from build123d import *

# Parameters (mm, degrees)
SKETCH1_R               = 9.64479785
BOSS_EXTRUDE1_DEPTH     = 1
SKETCH2_W               = 8
SKETCH2_H               = 8
SKETCH2_W_2             = 10
SKETCH2_H_2             = 10
SKETCH2_W_3             = 7
SKETCH2_H_3             = 7
BOSS_EXTRUDE2_DEPTH     = 9.5
SKETCH3_R               = 0.9
CUT_EXTRUDE1_DEPTH      = 8
CUT_EXTRUDE2_DEPTH      = 0.7
SKETCH6_R               = 6.717749006
CUT_EXTRUDE7_DEPTH      = 10.5
CUT_EXTRUDE7_DEPTH_BACK = 2


with BuildPart() as part:
    # Sketch1 → Boss-Extrude1 (new body)
    with BuildSketch(Plane.XY):
        with BuildLine():
            Line((-14.026724751, 23.745574299), (14.026724751, 23.745574299))
            ThreePointArc((14.026724751, 23.745574299), (37.77229905, 0), (14.026724751, -23.745574299))
            Line((14.026724751, -23.745574299), (-14.026724751, -23.745574299))
            ThreePointArc((-14.026724751, -23.745574299), (-37.77229905, 0), (-14.026724751, 23.745574299))
        make_face()
        Circle(SKETCH1_R, mode=Mode.SUBTRACT)
    extrude(amount=BOSS_EXTRUDE1_DEPTH)

    # Sketch2 → Boss-Extrude2 (add)
    with BuildSketch(Plane.XY.offset(1)):
        with Locations((-25.018703454, 11.462322744)):
            Rectangle(SKETCH2_W, SKETCH2_H)
        with Locations((-3.090198121, -14.497536266)):
            Rectangle(SKETCH2_W_2, SKETCH2_H_2)
        with Locations((25.327090693, 14.846915234)):
            Rectangle(SKETCH2_W_3, SKETCH2_H_3)
    extrude(amount=BOSS_EXTRUDE2_DEPTH)

    # Sketch3 → Cut-Extrude1 (cut)
    with BuildSketch(Plane.XY.offset(10.5)):
        with Locations((-25.018703454, 11.462322744)):
            Circle(SKETCH3_R)
        with Locations((25.327090693, 14.846915234)):
            Circle(SKETCH3_R)
        with Locations((-3.090198121, -14.497536266)):
            Circle(SKETCH3_R)
    extrude(amount=-CUT_EXTRUDE1_DEPTH, mode=Mode.SUBTRACT)

    # Sketch4 → Cut-Extrude2 (cut)
    with BuildSketch(Plane.XY.offset(1)):
        with BuildLine():
            Line((-20.6, 6.2), (-36.948598558, 6.2))
            ThreePointArc((-36.948598558, 6.2), (-37.70555704, 1.779100955), (-37.617693234, -2.705273523))
            Line((-37.617693234, -2.705273523), (-20.6, -2.705273523))
            Line((-20.6, -2.705273523), (-20.6, 6.2))
        make_face()
    extrude(amount=-CUT_EXTRUDE2_DEPTH, mode=Mode.SUBTRACT)

    # Sketch6 → Cut-Extrude7 (cut, two sides)
    with BuildSketch(Plane.XY.offset(1)) as cut_extrude7_sk:
        with Locations((14.176031791, 0)):
            Circle(SKETCH6_R)
        with Locations((-14.176031791, 0)):
            Circle(SKETCH6_R)
    extrude(amount=CUT_EXTRUDE7_DEPTH, mode=Mode.SUBTRACT)
    extrude(cut_extrude7_sk.sketch, amount=-CUT_EXTRUDE7_DEPTH_BACK, mode=Mode.SUBTRACT)


solid = part.part
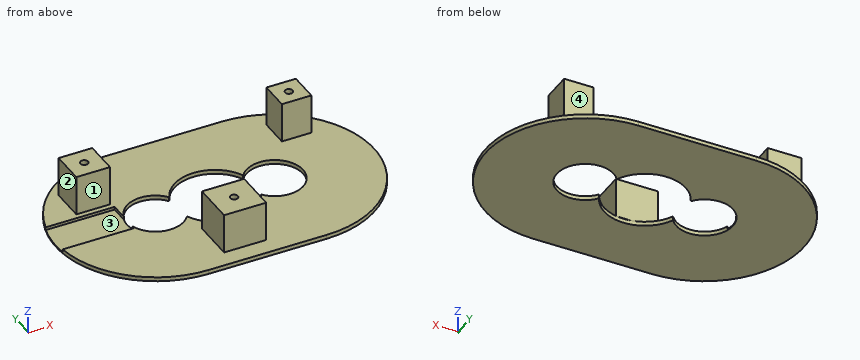
Work out the finished part from the listing and answer in its coordinate system (mm). Face numbers are marked on the shaded views. A direction names the side the tool comes from. Coordinates: 2 decimals unless noted, no trailing zeros. Loops run counter-clockwise (first coordinate to the right, second up) from the corner with the lowest first, then second, coordinate; pieces in that order, holes last. Notation, with made-up numbers: (36, -18) -> (84, -18) arc R14 cw to (84, -5) -> close; hole circle Ø2 at (-18.75, 68.5). An arc over 180 degrees is marked (long way). Write each question's results on one line, items separated by ' | '. Start each with the question number.
1) Find section B-B on y = 0. Determine the outline of the cut face in (x, z), then the cut area to 3 significant figures.
2) For the marked faces 1, 2, 3 and 4, determine the directions among +Z, -Z, +X, -X, +Y, -Y from which every point of the face is accessible in a straight line to the end or side of a thin tool.
3) Consider line 1 along Z through (x, y) = (1, 14); line 2 along X through (y, z) = (0, 0.8); line 3 along Y through (x, z) = (24, 5). Determine where each line is inside the solid, lowest interval first.
4) Find section C-C on x = -30. Determine the outline of the cut face in (y, z).
5) Find section D-D on y = -12.5. Determine the outline of the cut face in (x, z).
6) Flat-ended cylindrical pins translate along their axes: P1, Ø4, axis at x = -25, z = 7, coming from the -Y side; P2, Ø4, axis at x = 20, z = 5.5, coming from the -Y side; P3, Ø1.5, axis at y = -12, z = 8.5, coming from the +X side; P4, Ø4, axis at x = 24, y = -0.5, coming from the -Z side. Find the tip coordinate at first contact, or state that the pin passes through.
7) Find section A-A on z = 3.5. Determine the outline of the cut face in (x, y), then the cut area to 3 significant figures.
Response values:
1) outline: (-37.77, 0) -> (-20.89, 0) -> (-20.89, 0.3) -> (-37.77, 0.3) -> close; (20.89, 0) -> (37.77, 0) -> (37.77, 1) -> (20.89, 1) -> close | area: 21.9 mm^2
2) face 1: +Z, +X, -X, -Y | face 2: +Z, -X, +Y, -Y | face 3: +Z, -X | face 4: +Z, +X, -X, +Y
3) line 1: z = 0 to 1 | line 2: x = 20.89 to 37.77 | line 3: y = 11.35 to 18.35
4) outline: (-17.57, 0) -> (17.57, 0) -> (17.57, 1) -> (6.2, 1) -> (6.2, 0.3) -> (-2.71, 0.3) -> (-2.71, 1) -> (-17.57, 1) -> close
5) outline: (-34.22, 0) -> (34.22, 0) -> (34.22, 1) -> (1.91, 1) -> (1.91, 10.5) -> (-8.09, 10.5) -> (-8.09, 1) -> (-34.22, 1) -> close
6) P1: stops at y = 7.46 | P2: stops at y = 11.35 | P3: stops at x = 1.91 | P4: stops at z = 0
7) outline: (-29.02, 7.46) -> (-21.02, 7.46) -> (-21.02, 15.46) -> (-29.02, 15.46) -> close; (-8.09, -19.5) -> (1.91, -19.5) -> (1.91, -9.5) -> (-8.09, -9.5) -> close; (21.83, 11.35) -> (28.83, 11.35) -> (28.83, 18.35) -> (21.83, 18.35) -> close; hole circle Ø1.8 at (-25.02, 11.46); hole circle Ø1.8 at (-3.09, -14.5); hole circle Ø1.8 at (25.33, 14.85) | area: 205 mm^2
